Here's how the part is built. I have some questions about the finished solid (model axes, mm). A direction names the side the tool comes from. Round coordinates to 2 decimals unless told otherwise and drop trailing zeros. Order: outer loops, then holes, each group sorted by start corner. A loop starts at its lowest first (then second) coordinate and runs counter-clockwise, first axis right, second up. Notation, with made-up numbers: (-10.5, 18) - (18.5, 18) arc R32 ccw to (18.5, 53) - close; hole circle Ø1 at (56, -15.75). An arc over 180 degrees is marked (long way). Answer as a JSON object with one key per item and string values.
```python
from build123d import *

# Parameters (mm, degrees)
F0_W     = 26.8
F0_H     = 7.5
F1_DEPTH = 1.6
F2_W     = 5
F2_H     = 50.4
F2_H_2   = 4.5
F2_W_2   = 5.9
F2_H_3   = 4.3
F2_W_3   = 2.25
F2_H_4   = 7.5
F2_H_5   = 15.7
F3_DEPTH = 8.5
F4_W     = 7.5
F4_H     = 9.25
F5_DEPTH = 4
F6_W     = 5.05
F6_H     = 11.4
F7_DEPTH = 7.5
F8_R     = 1.6
F9_DEPTH = 5


with BuildPart() as f1:
    # F0 (on Top) → F1 (new body)
    with BuildSketch(Plane.XY):
        Polygon((0, 83.3), (0, 0), (48.2, 0), (48.2, 83.3), (37.5, 83.3), (10.7, 83.3), align=None)
        with Locations((24.1, 87.05)):
            Rectangle(F0_W, F0_H)
    extrude(amount=F1_DEPTH)

    # F2 (on face) → F3 (join)
    with BuildSketch(Plane.XY.offset(1.6)):
        with Locations((3.75, 49.9)):
            Rectangle(F2_W, F2_H)
        with Locations((44.45, 80.55)):
            Rectangle(F2_W, F2_H_2)
        with Locations((44.45, 49.9)):
            Rectangle(F2_W, F2_H)
        with Locations((5.05, 2.15)):
            Rectangle(F2_W_2, F2_H_3)
        with Locations((37.875, 55.05)):
            Rectangle(F2_W_3, F2_H_4)
        with Locations((3.75, 14.35)):
            Rectangle(F2_W, F2_H_5)
        with Locations((44.45, 14.35)):
            Rectangle(F2_W, F2_H_5)
    extrude(amount=F3_DEPTH)

    # F4 (on face) → F5 (join)
    with BuildSketch(Plane.XY.offset(1.6)):
        with Locations((24.9, 2.775)):
            Rectangle(F4_W, F4_H)
    extrude(amount=F5_DEPTH)

    # F6 (on face) → F7 (join)
    with BuildSketch(Plane.XY.offset(1.6)):
        with Locations((14.575, 3.65)):
            Rectangle(F6_W, F6_H)
    extrude(amount=F7_DEPTH)

    # F8 (on face) → F9 (join)
    with BuildSketch(Plane.XY.offset(1.6)):
        with Locations((3.85, 80)):
            Circle(F8_R)
    extrude(amount=F9_DEPTH)


solid = f1.part
```
1. If I drill on L1, parallel to Y at x = 45, z = 9; L2, parallel to X at y = 58, z = 7; L3, parallel to X at y = 69.5, z = 9.75, over which ranges is the centre line in solid material (lowest first)? Write a range as [from, to].
Responses:
{"L1": "[6.5, 22.2], [24.7, 75.1], [78.3, 82.8]", "L2": "[1.25, 6.25], [36.75, 39], [41.95, 46.95]", "L3": "[1.25, 6.25], [41.95, 46.95]"}
2. Imagine slicing it at B-B (x = 3.85). List the corners of the cut face in (y, z) for me, plus the area to 3 significant figures.
Responses:
{"outline": "(0, 0) - (83.3, 0) - (83.3, 1.6) - (81.6, 1.6) - (81.6, 6.6) - (78.4, 6.6) - (78.4, 1.6) - (75.1, 1.6) - (75.1, 10.1) - (24.7, 10.1) - (24.7, 1.6) - (22.2, 1.6) - (22.2, 10.1) - (6.5, 10.1) - (6.5, 1.6) - (4.3, 1.6) - (4.3, 10.1) - (0, 10.1) - close", "area": "748 mm2"}
3. Imagine slicing it at A-A (z = 7.5). Give the number of separate pieces and of enclosed holes in the cut face, plus the area to 3 significant figures.
Responses:
{"separate pieces": "8", "enclosed holes": "0", "area": "783 mm2"}
4. For P1, Ø2.5, axis at y = 39, z = 6.5, coming from the -X side; P2, Ø4, axis at x = 42.5, z = 4.5, coming from the -Y side; P3, Ø2, axis at y = 2, z = 4.5, coming from the -X side, each with a flat end and sliding along its axis, tell me the tip position at first contact or that it passes through.
Responses:
{"P1": "x = 1.25", "P2": "y = 6.5", "P3": "x = 2.1"}
5. For faces 1 (the face through (44, 6.5, 6)), 2 (the face through (15, 0, 1)), 3 (the face through (17.1, 4, 5)), 4 (the face through (4, 22.2, 6)), which set-ups out of +Z, -Z, +X, -X, +Y, -Y let a thin tool reach every point of the face, with its end or its side?
Responses:
{"face 1": "+Z, +X, -Y", "face 2": "-Z, -X, -Y", "face 3": "+Z, +Y, -Y", "face 4": "+Z, +X, -X"}
6. Imagine slicing it at C-C (y = 33.5). List the corners of the cut face in (x, z) for me.
Responses:
{"outline": "(0, 0) - (48.2, 0) - (48.2, 1.6) - (46.95, 1.6) - (46.95, 10.1) - (41.95, 10.1) - (41.95, 1.6) - (6.25, 1.6) - (6.25, 10.1) - (1.25, 10.1) - (1.25, 1.6) - (0, 1.6) - close"}
7. Thinking about a two-plate mould opening in X: for faces 5 (the face through (36.75, 55, 6)), 6 (the face through (2.1, 2, 6)), 7 (the face through (4, 24.7, 6)), which applies, pulls with the +X half, pulls with the -X half, needs draft (parallel to the pull), parting line crosses it, or undercut?
Responses:
{"face 5": "undercut", "face 6": "pulls with the -X half", "face 7": "needs draft"}
8. Imagine slicing it at D-D (x = 24.5). List the corners of the cut face in (y, z) for me.
Responses:
{"outline": "(-1.85, 1.6) - (0, 1.6) - (0, 0) - (90.8, 0) - (90.8, 1.6) - (7.4, 1.6) - (7.4, 5.6) - (-1.85, 5.6) - close"}
